from build123d import *

# Parameters (mm, degrees)
SKETCH1_R           = 39.5
BOSS_EXTRUDE1_DEPTH = 2
CIRPATTERN1_COUNT   = 3


with BuildPart() as part:
    # Sketch1 → Boss-Extrude1 (new body)
    with BuildSketch(Plane.XY):
        Circle(SKETCH1_R)
    extrude(amount=BOSS_EXTRUDE1_DEPTH)

    # Sketch3 → CSK for M4 Flat Head Machine Screw1 (revolve, cut)
    with BuildSketch(Plane(origin=(33, 0, 2), x_dir=(0, -1, 0), z_dir=(1, 0, 0))):
        Polygon((0, 0), (0, 27.391936393), (2.25, 26.04), (2.25, 2.45), (4.7, 0), align=None)
    csk_for_m4_flat_head_machine_screw1 = revolve(axis=Axis((33, 0, 8.35), (0, 0, -1)), mode=Mode.SUBTRACT)

    # CirPattern1: CSK for M4 Flat Head Machine Screw1 ×3 about axis
    cirpattern1_axis = Axis((0, 0, 0), (0, 0, 1))
    for i in range(1, CIRPATTERN1_COUNT):
        add(csk_for_m4_flat_head_machine_screw1.rotate(cirpattern1_axis, i * 360 / CIRPATTERN1_COUNT), mode=Mode.SUBTRACT)


solid = part.part
Input: part model. Units: mm. Frame: model coordinates. Give positions to 0.01 mm unless a question says otherwise; leave off trailing zeros. Write each loop counter-clockwise with the first axis right and the second up, starting at its lowest first coordinate (ties: lowest second). Pieces come first, ordered by that corner, then holes.
Q1. Section B-B, the plane x = 33. Output: boundary loops of the cut face in (y, z), plus the area to 3 significant figures.
Q2. Section C-C, the plane z = 0.35. Output: boundary loops of the cut face in (x, y).
Q3. Section D-D, the plane y = -9. Output: boundary loops of the cut face in (x, z), plus the area to 3 significant figures.
Q4. Material intervals for probe 1 along Y at (x, z) = (-18.5, 1); probe 2 along X at (y, z) = (28, 1.45); probe 3 along Y at (x, z) = (-0.5, 0.5), sorted ascending.
Q5. Section A-A, the plane x = -16.5. Output: boundary loops of the cut face in (y, z), plus the area to 3 significant figures.
Filled in:
1. outline: (-21.71, 0) - (-2.7, 0) - (-4.7, 2) - (-21.71, 2) - close; (2.7, 0) - (21.71, 0) - (21.71, 2) - (4.7, 2) - close
1. area: 72.0 mm2
2. outline: circle Ø79 at (0, 0); hole circle Ø6.1 at (-16.5, -28.58); hole circle Ø6.1 at (-16.5, 28.58); hole circle Ø6.1 at (33, 0)
3. outline: (-38.46, 0) - (38.46, 0) - (38.46, 2) - (-38.46, 2) - close
3. area: 154 mm2
4. probe 1: y = -34.9 to -31.69, -25.47 to 25.47, 31.69 to 34.9
4. probe 2: x = -27.86 to -20.61, -12.39 to 27.86
4. probe 3: y = -39.5 to 39.5
5. outline: (-35.89, 0) - (-31.28, 0) - (-33.28, 2) - (-35.89, 2) - close; (-25.88, 0) - (25.88, 0) - (23.88, 2) - (-23.88, 2) - close; (31.28, 0) - (35.89, 0) - (35.89, 2) - (33.28, 2) - close
5. area: 114 mm2
